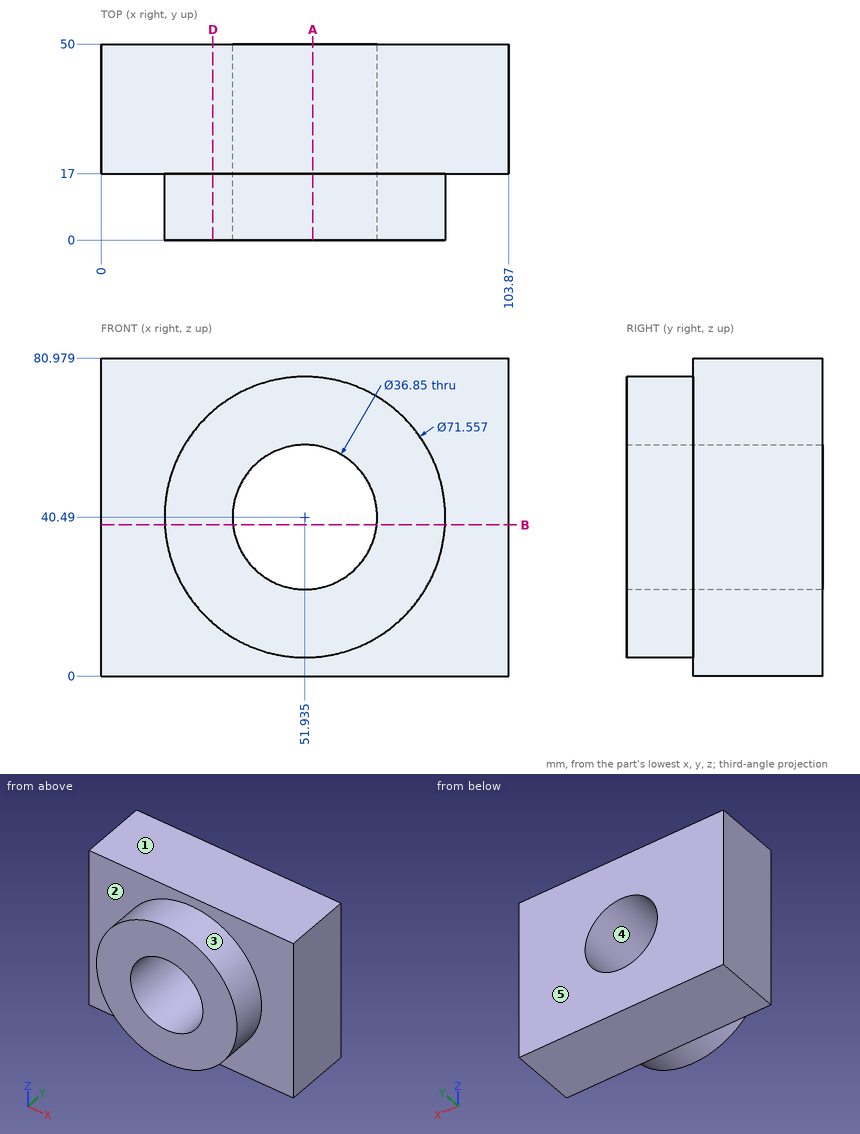
Part print with two shaded views. Sizes in mm from the minimum x, y, z corner. A direction names the side the tool comes from. Give positions to 0.01 mm unless a question says otherwise; leave off trailing zeros. Order: outer loops, then holes, each group sorted by start corner. A loop starts at its lowest first (then second) coordinate and runs counter-clockwise, first axis right, second up.
1) Saw through at A-A, the plane x = 54. Write the cut outline in (y, z), then the cut area to 3 significant figures.
2) Pin check, flat tips, straight feed: pin 1 (10 mm diameter, centred on y = 8, z = 14, fed in from -X); pin 2 (1 mm diameter, centred on x = 71, y = 8.5, fed in from +Z) (1 decimal). Stop position of each tip, or through.
3) Wall check: probe 1 along Y at (x, z) = (71, 75); probe 2 along X at (y, z) = (21.5, 41.5); probe 3 along Z at (x, y) = (40.5, 19.5) (1 decimal). Give the ranges that are in metal, low to high.
4) Saw through at B-B, the plane z = 38.5. Write the cut outline in (x, y).
5) 3-axis set-ups, long thin cutter, end or side, ignore diameter. For the marked faces 1 and 2: which of +Z, -Z, +X, -X, +Y, -Y reach the whole face in a straight line?
6) Saw through at D-D, the plane x = 28.5. Write the cut outline in (y, z) (1 decimal).
7) Mould opens along X. For the marked faces 3, 4 and 5 say: +X half, -X half, draft (parallel to the pull), parting line (faces both ways), or undercut.
Computed:
1. outline: (0, 4.77) - (17, 4.77) - (17, 0) - (50, 0) - (50, 22.18) - (0, 22.18) - close; (0, 58.8) - (50, 58.8) - (50, 80.98) - (17, 80.98) - (17, 76.21) - (0, 76.21) - close
1. area: 2,060 mm2
2. pin 1: stops at x = 23.33
2. pin 2: stops at z = 71.1
3. probe 1: y = 17 to 50
3. probe 2: x = 0 to 33.54, 70.33 to 103.87
3. probe 3: z = 0 to 26, 54.9 to 81
4. outline: (0, 17) - (16.21, 17) - (16.21, 0) - (33.62, 0) - (33.62, 50) - (0, 50) - close; (70.25, 0) - (87.66, 0) - (87.66, 17) - (103.87, 17) - (103.87, 50) - (70.25, 50) - close
5. face 1: +Z, +X, -X, +Y, -Y
5. face 2: -Y
6. outline: (0, 13.5) - (17, 13.5) - (17, 0) - (50, 0) - (50, 81) - (17, 81) - (17, 67.5) - (0, 67.5) - close
7. face 3: parting line
7. face 4: undercut
7. face 5: draft
